Design review of the part built by this model. Coordinates are the model's own, in mm. Give positions to 0.01 mm unless a question says otherwise; leave off trailing zeros. Loops run counter-clockwise (first coordinate to the right, second up) from the corner with the lowest first, then second, coordinate; pieces in that order, holes last. Notation, with made-up numbers: M 21.25,85 L 56.25,85 A28 cw 56.25,113 Z; hole C -22,15 d11. An arc over 180 degrees is marked long. Use one line per item in the form item = value. Start each with the question number.
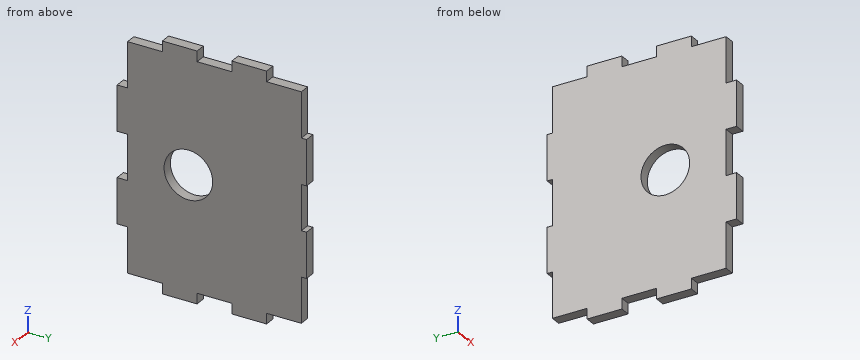
from build123d import *

# Parameters (mm, degrees)
SKETCH1_R           = 14
BOSS_EXTRUDE1_DEPTH = 6


with BuildPart() as part:
    # Sketch1 → Boss-Extrude1 (new body)
    with BuildSketch(Plane(origin=(0, 0, 0), x_dir=(0, 0, -1), z_dir=(1, 0, 0))):
        Polygon((65, -30), (71, -30), (71, -10), (65, -10), (65, 10), (71, 10), (71, 30), (65, 30), (65, 50), (39, 50), (39, 53), (13, 53), (13, 50), (-13, 50), (-13, 53), (-39, 53), (-39, 50), (-65, 50), (-65, 30), (-71, 30), (-71, 10), (-65, 10), (-65, -10), (-71, -10), (-71, -30), (-65, -30), (-65, -50), (-39, -50), (-39, -56), (-13, -56), (-13, -50), (13, -50), (13, -56), (39, -56), (39, -50), (65, -50), align=None)
        with Locations((0, -15)):
            Circle(SKETCH1_R, mode=Mode.SUBTRACT)
    extrude(amount=BOSS_EXTRUDE1_DEPTH)


solid = part.part
Q1. Take a section at D-D on y = -47. Give the boundary of the cut face in (x, z).
Q2. Take a section at C-C on z = 59.5. Give the boundary of the cut face in (x, y).
Q3. Clearance check with flat-ended pins moving along their axes: pin 1 Ø3 at (x, z) = (2, 12.5) entering from +Y; pin 2 Ø3 at (x, y) = (3.5, -54.5) entering from -Z; pin 3 Ø3 at (x, y) = (3, 0.5) entering from +Z; pin 4 Ø1.8 at (x, z) = (3, 68.5) entering from +Y. State where each tip first meets the part, or that it passes through.
Q4. Take a section at A-A on y = -15. Give the boundary of the cut face in (x, z).
Q5. Take a section at B-B on z = 0. Give the boundary of the cut face in (x, y), plus the area to 3 significant figures.
Q6. Wall thickness on probe 1 along Y at (x, z) = (1.6, 0); probe 2 along Z at (x, y) = (4.7, -32); probe 3 along Y at (x, z) = (3.05, 46): over which ranges is each line inside the solid? List them lowest first.
Response values:
q1.outline = M 0,-65 L 6,-65 L 6,65 L 0,65 Z
q2.outline = M 0,-50 L 6,-50 L 6,50 L 0,50 Z
q3.pin_1 = 53
q3.pin_2 = -39
q3.pin_3 = 65
q3.pin_4 = 30
q4.outline = M 0,-71 L 6,-71 L 6,-14 L 0,-14 Z; M 0,14 L 6,14 L 6,71 L 0,71 Z
q5.outline = M 0,-50 L 6,-50 L 6,-29 L 0,-29 Z; M 0,-1 L 6,-1 L 6,50 L 0,50 Z
q5.area = 432 mm^2
q6.probe_1 = -50 to -29, -1 to 50
q6.probe_2 = -65 to 65
q6.probe_3 = -50 to 50
